from build123d import *

# Parameters (mm, degrees)
SKETCH_2_R               = 1.75
EXTRUDE_1_DEPTH          = 8
CUT_EXTRUDE_1_DEPTH      = 40.940580867
CUT_EXTRUDE_1_DEPTH_BACK = 40.940580867
CUT_EXTRUDE_2_DEPTH      = 3.5
CUT_EXTRUDE_2_DEPTH_BACK = 3.5
SKETCH_6_R               = 3.25


with BuildPart() as part:
    # Sketch 2 → Extrude 1 (new body)
    with BuildSketch(Plane(origin=(0, 0, 0), x_dir=(-1, 0, 0), z_dir=(0, 1, 0))):
        with BuildLine():
            Line((5, -17.5), (-5, -17.5))
            Line((-5, -17.5), (-15.5, -17.5))
            ThreePointArc((-15.5, -17.5), (-16.914213562, -16.914213562), (-17.5, -15.5))
            Line((-17.5, -15.5), (-17.5, 15.5))
            ThreePointArc((-17.5, 15.5), (-16.914213562, 16.914213562), (-15.5, 17.5))
            Line((-15.5, 17.5), (-5, 17.5))
            Line((-5, 17.5), (5, 17.5))
            Line((5, 17.5), (15.5, 17.5))
            ThreePointArc((15.5, 17.5), (16.914213562, 16.914213562), (17.5, 15.5))
            Line((17.5, 15.5), (17.5, -15.5))
            ThreePointArc((17.5, -15.5), (16.914213562, -16.914213562), (15.5, -17.5))
            Line((15.5, -17.5), (5, -17.5))
        make_face()
        with Locations(Location((10, 0, 0), (0, 0, 90))):
            Circle(SKETCH_2_R, mode=Mode.SUBTRACT)
        with Locations(Location((-10, 0, 0), (0, 0, 90))):
            Circle(SKETCH_2_R, mode=Mode.SUBTRACT)
    extrude(amount=EXTRUDE_1_DEPTH)

    # Sketch 4 → Cut-Extrude 1 (cut, two sides: drawn at the far end of the back side and taken through both)
    with BuildSketch(Plane.XY.offset(17.5).offset(-CUT_EXTRUDE_1_DEPTH_BACK)):
        with BuildLine():
            Line((-98.814506181, 16.947453844), (-17.5, 8))
            ThreePointArc((-17.5, 8), (0, 7.040089286), (17.5, 8))
            Line((17.5, 8), (98.814506181, 16.947453844))
            Line((98.814506181, 16.947453844), (98.814506181, 180.558038412))
            Line((98.814506181, 180.558038412), (-98.814506181, 180.558038412))
            Line((-98.814506181, 180.558038412), (-98.814506181, 16.947453844))
        make_face()
    extrude(amount=CUT_EXTRUDE_1_DEPTH + CUT_EXTRUDE_1_DEPTH_BACK, mode=Mode.SUBTRACT)

    # Sketch 6 → Cut-Extrude 2 (cut, two sides: drawn at the far end of the back side and taken through both)
    with BuildSketch(Plane(origin=(0, 7.352932668, 0), x_dir=(-1, 0, 0), z_dir=(0, -1, 0)).offset(-CUT_EXTRUDE_2_DEPTH_BACK)):
        with Locations(Location((10, 0, 0), (0, 0, 90))):
            Circle(SKETCH_6_R)
        with Locations(Location((-10, 0, 0), (0, 0, 90))):
            Circle(SKETCH_6_R)
    extrude(amount=CUT_EXTRUDE_2_DEPTH + CUT_EXTRUDE_2_DEPTH_BACK, mode=Mode.SUBTRACT)


solid = part.part
Could you check a few things on this model? Use its own coordinates, in mm. A direction names the side the tool comes from. Give positions to 0.01 mm unless a question says otherwise; leave off trailing zeros. Order: outer loops, then holes, each group sorted by start corner. A loop starts at its lowest first (then second) coordinate and runs counter-clockwise, first axis right, second up. Notation, with made-up numbers: (-13.5, -21) - (-9.5, -21) arc R19 ccw to (-9.5, -16) - close; hole circle Ø3 at (-13, 67.5). An arc over 180 degrees is marked (long way). One line per item, written item: value. Start each with the question number.
1. For P1, Ø2, axis at x = 8.5, z = 1.5, coming from the +Y side; P2, Ø10, axis at x = 1, z = 9.5, coming from the +Y side; P3, Ø5, axis at x = -10, z = 0, coming from the -Y side; P4, Ø8.5, axis at x = 10, z = 0, coming from the +Y side, each with a flat end and sliding along its axis, tell me the tip position at first contact or that it passes through.
2. Imagine slicing it at B-B on x = -10. List the corners of the cut face in (y, z) for me.
3. If I drill on probe 1 along X at (y, z) = (5.8, 0); probe 2 along X at (y, z) = (3.25, -1); probe 3 along Z at (x, y) = (-10, 5.5), over which ranges is the centre line in solid material (lowest first)?
4. Imagine slicing it at A-A on y = 4.75. List the corners of the cut face in (x, z) for me.
5. Imagine slicing it at C-C on z = 0. List the corners of the cut face in (x, y) for me, plus the area to 3 significant figures.
6. Thinking about a two-plate mould opening in X: for faces 1 (the face through (-11.4, 3.853, -1.4)), 2 (the face through (-12.883, 5.75, -1.5)), 3 (the face through (-17.5, 4, 0)), 4 (the face through (0, 4, 17.5)), which applies, +X half, -X half, draft (parallel to the pull), parting line (faces both ways), or undercut?
7. Imagine slicing it at D-D on y = 1. List the corners of the cut face in (x, z) for me.
8. For faces 5 (the face through (8.6, 3.853, -1.4)), 6 (the face through (-0.25, 7.04, -0.25)), which set-ups out of +Z, -Z, +X, -X, +Y, -Y let a thin tool reach every point of the face, with its end or its side?
Values:
1. P1: y = 3.85
1. P2: y = 7.15
1. P3: y = 0
1. P4: y = 7.68
2. outline: (0, -17.5) - (7.35, -17.5) - (7.35, -3.25) - (3.85, -3.25) - (3.85, -1.75) - (0, -1.75) - close; (0, 1.75) - (3.85, 1.75) - (3.85, 3.25) - (7.35, 3.25) - (7.35, 17.5) - (0, 17.5) - close
3. probe 1: -17.5 to -13.25, -6.75 to 6.75, 13.25 to 17.5
3. probe 2: -17.5 to -11.44, -8.56 to 8.56, 11.44 to 17.5
3. probe 3: -17.5 to -3.25, 3.25 to 17.5
4. outline: (-17.5, -15.5) arc R2 ccw to (-15.5, -17.5) - (15.5, -17.5) arc R2 ccw to (17.5, -15.5) - (17.5, 15.5) arc R2 ccw to (15.5, 17.5) - (-15.5, 17.5) arc R2 ccw to (-17.5, 15.5) - close; hole circle Ø6.5 at (-10, 0); hole circle Ø6.5 at (10, 0)
5. outline: (-17.5, 0) - (-11.75, 0) - (-11.75, 3.85) - (-13.25, 3.85) - (-13.25, 7.59) arc R160 cw to (-17.5, 8) - close; (-8.25, 0) - (8.25, 0) - (8.25, 3.85) - (6.75, 3.85) - (6.75, 7.18) arc R160 cw to (-6.75, 7.18) - (-6.75, 3.85) - (-8.25, 3.85) - close; (11.75, 0) - (17.5, 0) - (17.5, 8) arc R160 cw to (13.25, 7.59) - (13.25, 3.85) - (11.75, 3.85) - close
5. area: 185 mm²
6. face 1: undercut
6. face 2: undercut
6. face 3: -X half
6. face 4: draft
7. outline: (-17.5, -15.5) arc R2 ccw to (-15.5, -17.5) - (15.5, -17.5) arc R2 ccw to (17.5, -15.5) - (17.5, 15.5) arc R2 ccw to (15.5, 17.5) - (-15.5, 17.5) arc R2 ccw to (-17.5, 15.5) - close; hole circle Ø3.5 at (-10, 0); hole circle Ø3.5 at (10, 0)
8. face 5: +Y
8. face 6: +Z, -Z, +Y
